Part model, mm, in its own coordinate system. A direction names the side the tool comes from. Give positions to 0.01 mm unless a question says otherwise; leave off trailing zeros. Order: outer loops, then holes, each group sorted by start corner. A loop starts at its lowest first (then second) coordinate and runs counter-clockwise, first axis right, second up. Notation, with made-up numbers: M 63.25,68 L 114.25,68 A31 cw 114.25,95 Z; hole C 51.5,76 d1. An arc over 180 degrees is marked long. Return JSON: item names as keys, results as strings.
from build123d import *

# Parameters (mm, degrees)
F0_R     = 10
F0_R_2   = 7.5
F1_DEPTH = 120
F2_DEPTH = 15.1
F3_D     = 6.8
F3_DEPTH = 45
F3_TIP   = 2.0429261047
F4_SIZE  = 0.3


with BuildPart() as f1:
    # F0 (on Top) → F1 (new body)
    with BuildSketch(Plane.XY):
        Circle(F0_R)
        Circle(F0_R_2, mode=Mode.SUBTRACT)
        Circle(F0_R_2)
    extrude(amount=F1_DEPTH)

    # F0 (on Top) → F2 (cut)
    with BuildSketch(Plane.XY):
        Circle(F0_R_2)
    extrude(amount=F2_DEPTH, mode=Mode.SUBTRACT)

    # F3
    with Locations(Plane(origin=(0, 0, 0), x_dir=(1, 0, 0), z_dir=(0, 0, -1))):
        with Locations((0, 0)):
            Hole(F3_D / 2, depth=F3_DEPTH)
            with Locations((0, 0, -(F3_DEPTH + F3_TIP / 2))):  # 118° drill point
                Cone(0, F3_D / 2, F3_TIP, mode=Mode.SUBTRACT)

    # F4
    f4_edges = [f1.edges().sort_by_distance(p)[0] for p in [
        (-10, 0, 120),
        (-7.5, 0, 0),
        (-10, 0, 0),
    ]]
    chamfer(f4_edges, length=F4_SIZE)


solid = f1.part
Q1. Band-saw the part on A-A (z = 34.5). Give the cut face in (x, y).
Established:
{"outline": "C 0,0 d20; hole C 0,0 d6.8"}
Q2. Band-saw the part on B-B (z = 108.5). Give the cut face in (x, y).
Established:
{"outline": "C 0,0 d20"}
Q3. 3-axis set-ups, long thin cutter, end or side, ignore diameter. For faces 1 (the flat face through (2, -3, 15.1)), 2 (the flat face through (0, 0, 120)): which of +Z, -Z, +X, -X, +Y, -Y reach the whole face in a straight line?
Established:
{"face 1": "-Z", "face 2": "+Z, +X, -X, +Y, -Y"}
Q4. Two-plate mould, pull along X, no slides. Class faces 3 (the cylindrical face through (-2.17, -9.76, 59.16)), 4 (the flat face through (-7, 4, 0)), 5 (the cylindrical face through (-7.493, 0.33, 7.596)): +X half, -X half, draft (parallel to the pull), parting line (faces both ways), or undercut.
Established:
{"face 3": "parting line", "face 4": "draft", "face 5": "undercut"}
Q5. Probe line 1 along Y through (x, z) = (0, 34.75); line 2 along Y through (x, z) = (0, 6.75); line 3 along Z through (x, y) = (-2.75, -3.75). List the from-to ranges inside material, lowest first.
Established:
{"line 1": "y = -10 to -3.4, 3.4 to 10", "line 2": "y = -10 to -7.5, 7.5 to 10", "line 3": "z = 15.1 to 120"}
Q6. Pin check, flat tips, straight feed: pin 1 (2 mm diameter, centred on y = 6.5, z = 25, fed in from +X); pin 2 (5 mm diameter, centred on y = 8, z = 74.5, fed in from -X); pin 3 (1.5 mm diameter, centred on x = 6.5, z = 97.5, fed in from +Y). Stop position of each tip, or through.
Established:
{"pin 1": "stops at x = 8.35", "pin 2": "stops at x = -8.35", "pin 3": "stops at y = 8.18"}
